Build history of the part. All positions in model axes, mm. Face numbers are marked on the shaded views. A direction names the side the tool comes from. Give positions to 0.01 mm unless a question says otherwise; leave off trailing zeros. Loops run counter-clockwise (first coordinate to the right, second up) from the corner with the lowest first, then second, coordinate; pieces in that order, holes last. Notation, with made-up numbers: (-6.5, 19.5) -> (-1.5, 19.5) arc R11 ccw to (-1.5, 27.5) -> close; hole circle Ø2 at (20.5, 52.5). An arc over 180 degrees is marked (long way). Answer in a Markdown table with one row per item. Add a question column.
from build123d import *

# Parameters (mm, degrees)
F1_DEPTH  = 3
F2_W      = 32
F2_H      = 4.25
F3_DEPTH  = 15
F4_W      = 32
F4_H      = 3
F5_DEPTH  = 27.75
F6_W      = 2
F6_H      = 1.8
F7_DEPTH  = 23.5
F8_W      = 4.25
F8_H      = 1.8
F9_DEPTH  = 5
F10_W     = 11
F10_H     = 5.8846425861
F11_DEPTH = 3


with BuildPart() as f1:
    # F0 (on Top) → F1 (new body)
    with BuildSketch(Plane.XY):
        Polygon((11.75, 11.75), (11.75, -11.75), (-11.75, -11.75), (-11.75, 11.75), (-16, 11.75), (-16, -16), (16, -16), (16, 11.75), align=None)
    extrude(amount=F1_DEPTH)

    # F2 (on face) → F3 (join)
    with BuildSketch(Plane(origin=(0, 0, 0), x_dir=(1, 0, 0), z_dir=(0, 0, -1))):
        with Locations((0, 13.875)):
            Rectangle(F2_W, F2_H)
    extrude(amount=F3_DEPTH)

    # F4 (on face) → F5 (join, through all)
    with BuildSketch(Plane.XZ.offset(16)):
        with Locations((0, -16.5)):
            Rectangle(F4_W, F4_H)
    extrude(amount=-F5_DEPTH)

    # F6 (on face) → F7 (cut, through all)
    with BuildSketch(Plane(origin=(0, 11.75, 0), x_dir=(-1, 0, 0), z_dir=(0, 1, 0))):
        with Locations((13.95, 0.9)):
            Rectangle(F6_W, F6_H)
        with Locations((-13.95, 0.9)):
            Rectangle(F6_W, F6_H)
    extrude(amount=-F7_DEPTH, mode=Mode.SUBTRACT)

    # F8 (on face) → F9 (cut)
    with BuildSketch(Plane(origin=(0, 11.75, 0), x_dir=(-1, 0, 0), z_dir=(0, 1, 0))):
        with Locations((-13.875, 0.9)):
            Rectangle(F8_W, F8_H)
    extrude(amount=-F9_DEPTH, mode=Mode.SUBTRACT)

    # F10 (on face) → F11 (cut, through all)
    with BuildSketch(Plane.XY.offset(-15)):
        with Locations((0, 8.8076787069)):
            Rectangle(F10_W, F10_H)
    extrude(amount=-F11_DEPTH, mode=Mode.SUBTRACT)


solid = f1.part
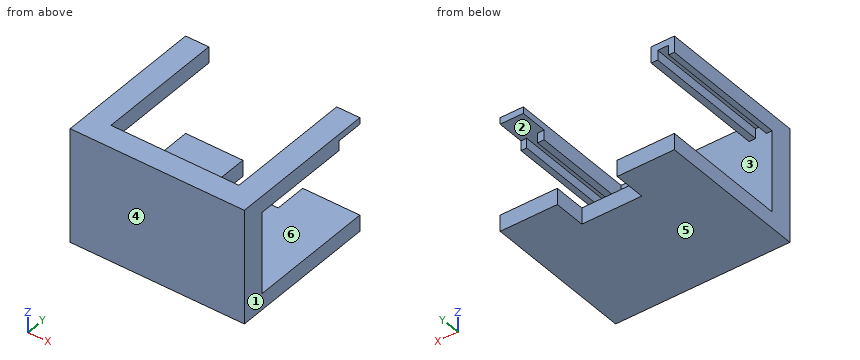
(1) Saw through at A-A, the plane y = 9. List the corners of the cut face in (x, z), then the cut area to 4 significant figures.
(2) Saw through at D-D, the plane x = -2. List the corners of the cut face in (y, z).
(3) 3-axis set-ups, long thin cutter, end or side, ignore diameter. For the marked faces 1 and 2: which of +Z, -Z, +X, -X, +Y, -Y reach the whole face in a straight line?
(4) Wall check: line 1 along X through (y, z) = (-5.5, 1); line 2 along X through (y, z) = (6.5, -16.5); line 3 along Y through (x, z) = (5, -16.25). Give the ranges that are in metal, low to high. Write a range as from..to.
(5) Two-plate mould, pull along Z, no slides. Class the marked faces 3, 4, 5 and 6: released by +Z, released by -Z, zero draft, split by the parting line, or undercut.
(6) Saw through at C-C, the plane z = -16.25. List the corners of the cut face in (x, y).
(7) Saw through at B-B, the plane y = 0. List the corners of the cut face in (x, z), then the cut area to 3 significant figures.
(8) Flat gauge pins, fed straight in: pin 1 Ø5 at (x, z) = (8, -0.5) entering from +Y; pin 2 Ø0.9 at (x, z) = (-2.5, -16) entering from +Y; pin 3 Ø0.5 at (x, z) = (15.5, 1) entering from +Y. Where does each tip first touch, or does it go through?
Worked answers:
| question | item | result |
|---|---|---|
| 1 | outline | (-16, -18) -> (-5.5, -18) -> (-5.5, -15) -> (-16, -15) -> close; (-16, 0) -> (-14.95, 0) -> (-14.95, 1.8) -> (-12.95, 1.8) -> (-12.95, 0) -> (-11.75, 0) -> (-11.75, 3) -> (-16, 3) -> close; (5.5, -18) -> (16, -18) -> (16, -15) -> (5.5, -15) -> close; (11.75, 1.8) -> (16, 1.8) -> (16, 3) -> (11.75, 3) -> close |
| 1 | area | 77.25 mm^2 |
| 2 | outline | (-16, -18) -> (5.87, -18) -> (5.87, -15) -> (-11.75, -15) -> (-11.75, 3) -> (-16, 3) -> close |
| 3 | face 1 | +Z, -Z, +X, +Y, -Y |
| 3 | face 2 | +Y |
| 4 | line 1 | -16..-14.95, -12.95..-11.75, 11.75..12.95, 14.95..16 |
| 4 | line 2 | -16..-5.5, 5.5..16 |
| 4 | line 3 | -16..5.87 |
| 5 | face 3 | undercut |
| 5 | face 4 | zero draft |
| 5 | face 5 | released by -Z |
| 5 | face 6 | undercut |
| 6 | outline | (-16, -16) -> (16, -16) -> (16, 11.75) -> (5.5, 11.75) -> (5.5, 5.87) -> (-5.5, 5.87) -> (-5.5, 11.75) -> (-16, 11.75) -> close |
| 7 | outline | (-16, -18) -> (16, -18) -> (16, -15) -> (-16, -15) -> close; (-16, 0) -> (-14.95, 0) -> (-14.95, 1.8) -> (-12.95, 1.8) -> (-12.95, 0) -> (-11.75, 0) -> (-11.75, 3) -> (-16, 3) -> close; (11.75, 0) -> (12.95, 0) -> (12.95, 1.8) -> (14.95, 1.8) -> (14.95, 0) -> (16, 0) -> (16, 3) -> (11.75, 3) -> close |
| 7 | area | 114 mm^2 |
| 8 | pin 1 | y = -11.75 |
| 8 | pin 2 | y = 5.87 |
| 8 | pin 3 | y = 6.75 |
